```python
from build123d import *

# Parameters (mm, degrees)
SKETCH1_R                                      = 38.1
BOSS_EXTRUDE1_DEPTH                            = 6.35
CBORE_FOR_4_BUTTON_HEAD_CAP_SCREW1_D           = 2.8702
CBORE_FOR_4_BUTTON_HEAD_CAP_SCREW1_CBORE_D     = 4.826
CBORE_FOR_4_BUTTON_HEAD_CAP_SCREW1_CBORE_DEPTH = 1.905
CIRPATTERN1_COUNT                              = 8
SKETCH6_R                                      = 0.396875
CUT_EXTRUDE1_DEPTH                             = 55.254423783
CIRPATTERN2_COUNT                              = 4
SKETCH7_R                                      = 0.79375


with BuildPart() as part:
    # Sketch1 → Boss-Extrude1 (new body)
    with BuildSketch(Plane(origin=(0, 0, 0), x_dir=(1, 0, 0), z_dir=(0, 1, 0))):
        with Locations(Location((0, 0, 0), (0, 0, 270))):
            Circle(SKETCH1_R)
    extrude(amount=BOSS_EXTRUDE1_DEPTH)

    # CBORE for #4 Button Head Cap Screw1 (through all)
    with Locations(Plane(origin=(0, 0, 0), x_dir=(-1, 0, 0), z_dir=(0, -1, 0))):
        with Locations((0, -33.3375)):
            cbore_for_4_button_head_cap_screw1 = CounterBoreHole(CBORE_FOR_4_BUTTON_HEAD_CAP_SCREW1_D / 2, CBORE_FOR_4_BUTTON_HEAD_CAP_SCREW1_CBORE_D / 2, CBORE_FOR_4_BUTTON_HEAD_CAP_SCREW1_CBORE_DEPTH)

    # CirPattern1: CBORE for #4 Button Head Cap Screw1 ×8 about axis
    cirpattern1_axis = Axis((0, 0, 0), (0, 1, 0))
    for i in range(1, CIRPATTERN1_COUNT):
        add(cbore_for_4_button_head_cap_screw1.rotate(cirpattern1_axis, i * 360 / CIRPATTERN1_COUNT), mode=Mode.SUBTRACT)

    # Sketch6 → Cut-Extrude1 (cut, through all)
    with BuildSketch(Plane.XZ):
        with Locations(Location((-0.644070231, -1.381213067, 0), (0, 0, 270))):
            Circle(SKETCH6_R)
        with Locations(Location((-1.381213067, -0.644070231, 0), (0, 0, 270))):
            Circle(SKETCH6_R)
    cut_extrude1 = extrude(amount=-CUT_EXTRUDE1_DEPTH, mode=Mode.SUBTRACT)

    # CirPattern2: Cut-Extrude1 ×4 about axis
    cirpattern2_axis = Axis((0.000227094, 0, 0.000227094), (0, 1, 0))
    for i in range(1, CIRPATTERN2_COUNT):
        add(cut_extrude1.rotate(cirpattern2_axis, i * 360 / CIRPATTERN2_COUNT), mode=Mode.SUBTRACT)

    # Cut-Sweep1: sweep along a curve in space
    with BuildLine() as cut_sweep1_path:
        Line((0, 6.35, -8.001), (0, 0, -6.35))
    # Sketch7 → Cut-Sweep1 (sweep, cut)
    with BuildSketch(Plane(origin=(0, 6.35, 0), x_dir=(1, 0, 0), z_dir=(0, 1, 0))):
        with Locations((0, 8.001)):
            Circle(SKETCH7_R)
    sweep(path=cut_sweep1_path.line, mode=Mode.SUBTRACT)

    # CirPattern3: read off the stored shape, not the designer's step
    # CirPattern3: loft between two sections, ruled curve by curve
    cirpattern3_from = [
        Edge.make_bspline([(-7.470778066, 7.350046313, 0.003515494), (-7.470778066, 7.350046313, -1.583984506), (-9.058278066, 7.350046313, -1.583984506), (-9.058278066, 7.350046313, 0.003515494), (-9.058278066, 7.350046313, 1.591015494), (-7.470778066, 7.350046313, 1.591015494), (-7.470778066, 7.350046313, 0.003515494)], [0, 0, 0, 0, 0.5, 0.5, 0.5, 1, 1, 1, 1], 3, [1, 0.333333333, 0.333333333, 1, 0.333333333, 0.333333333, 1]),
    ]
    cirpattern3_to = [
        Edge.make_bspline([(-5.299753984, -1.000046313, 0.003515494), (-5.299753984, -1.000046313, -1.583984506), (-6.887253984, -1.000046313, -1.583984506), (-6.887253984, -1.000046313, 0.003515494), (-6.887253984, -1.000046313, 1.591015494), (-5.299753984, -1.000046313, 1.591015494), (-5.299753984, -1.000046313, 0.003515494)], [0, 0, 0, 0, 0.5, 0.5, 0.5, 1, 1, 1, 1], 3, [1, 0.333333333, 0.333333333, 1, 0.333333333, 0.333333333, 1]),
    ]
    cirpattern3 = Solid(Shell([*[Face.make_surface_from_curves(cirpattern3_from[k], cirpattern3_to[k]) for k in range(1)], Face(Wire(cirpattern3_from)), Face(Wire(cirpattern3_to))]))
    add(cirpattern3, mode=Mode.SUBTRACT)

    # CirPattern3 2: loft between two sections, ruled curve by curve
    cirpattern3_2_from = [
        Edge.make_bspline([(-5.31e-07, 7.350046313, 7.474293561), (-1.587500531, 7.350046313, 7.474293561), (-1.587500531, 7.350046313, 9.061793561), (-5.31e-07, 7.350046313, 9.061793561), (1.587499469, 7.350046313, 9.061793561), (1.587499469, 7.350046313, 7.474293561), (-5.31e-07, 7.350046313, 7.474293561)], [0, 0, 0, 0, 0.5, 0.5, 0.5, 1, 1, 1, 1], 3, [1, 0.333333333, 0.333333333, 1, 0.333333333, 0.333333333, 1]),
    ]
    cirpattern3_2_to = [
        Edge.make_bspline([(-5.31e-07, -1.000046313, 5.303269478), (-1.587500531, -1.000046313, 5.303269478), (-1.587500531, -1.000046313, 6.890769478), (-5.31e-07, -1.000046313, 6.890769478), (1.587499469, -1.000046313, 6.890769478), (1.587499469, -1.000046313, 5.303269478), (-5.31e-07, -1.000046313, 5.303269478)], [0, 0, 0, 0, 0.5, 0.5, 0.5, 1, 1, 1, 1], 3, [1, 0.333333333, 0.333333333, 1, 0.333333333, 0.333333333, 1]),
    ]
    cirpattern3_2 = Solid(Shell([*[Face.make_surface_from_curves(cirpattern3_2_from[k], cirpattern3_2_to[k]) for k in range(1)], Face(Wire(cirpattern3_2_from)), Face(Wire(cirpattern3_2_to))]))
    add(cirpattern3_2, mode=Mode.SUBTRACT)

    # CirPattern3 3: loft between two sections, ruled curve by curve
    cirpattern3_3_from = [
        Edge.make_bspline([(7.470777536, 7.350046313, 0.003516025), (7.470777536, 7.350046313, 1.591016025), (9.058277536, 7.350046313, 1.591016025), (9.058277536, 7.350046313, 0.003516025), (9.058277536, 7.350046313, -1.583983975), (7.470777536, 7.350046313, -1.583983975), (7.470777536, 7.350046313, 0.003516025)], [0, 0, 0, 0, 0.5, 0.5, 0.5, 1, 1, 1, 1], 3, [1, 0.333333333, 0.333333333, 1, 0.333333333, 0.333333333, 1]),
    ]
    cirpattern3_3_to = [
        Edge.make_bspline([(5.299753453, -1.000046313, 0.003516025), (5.299753453, -1.000046313, 1.591016025), (6.887253453, -1.000046313, 1.591016025), (6.887253453, -1.000046313, 0.003516025), (6.887253453, -1.000046313, -1.583983975), (5.299753453, -1.000046313, -1.583983975), (5.299753453, -1.000046313, 0.003516025)], [0, 0, 0, 0, 0.5, 0.5, 0.5, 1, 1, 1, 1], 3, [1, 0.333333333, 0.333333333, 1, 0.333333333, 0.333333333, 1]),
    ]
    cirpattern3_3 = Solid(Shell([*[Face.make_surface_from_curves(cirpattern3_3_from[k], cirpattern3_3_to[k]) for k in range(1)], Face(Wire(cirpattern3_3_from)), Face(Wire(cirpattern3_3_to))]))
    add(cirpattern3_3, mode=Mode.SUBTRACT)


solid = part.part
```
Input: part model. Units: mm. Frame: model coordinates. A direction names the side the tool comes from. Give positions to 0.01 mm unless a question says otherwise; leave off trailing zeros. Order: outer loops, then holes, each group sorted by start corner. A loop starts at its lowest first (then second) coordinate and runs counter-clockwise, first axis right, second up.
1. Cut plane C-C (y = 4.25). State how many separate pieces and enclosed holes the cut face has, and give its area (3 significant figures).
Computed:
separate pieces: 1
enclosed holes: 20
area: 4,500 mm2
2. Line query: probe 1 along Z at (x, y) = (1.5, 2.5); probe 2 along Z at (x, y) = (-32.5, 5.5); probe 3 along X at (y, z) = (4.25, 23.5). Output: solid intervals per line, ascending.
Computed:
probe 1: z = -38.07 to -1.02, -0.27 to 0.27, 1.02 to 38.07
probe 2: z = -19.88 to -1.17, 1.17 to 19.88
probe 3: x = -29.99 to -25.01, -22.14 to 22.14, 25.01 to 29.99
3. Cut plane B-B (z = 29.5). Return loops of the section in (x, y), and give its area (3 significant figures).
Computed:
outline: (-24.11, 0) - (24.11, 0) - (24.11, 6.35) - (-24.11, 6.35) - close
area: 306 mm2
4. Set-up query: faces 1 (the face through (-33, 1.905, -2)), 2 (the face through (34.74, 4.16, 0.31)). Return all of +Z, -Z, +X, -X, +Y, -Y with unobstructed straight access to the full face (end or side cutting, diameter ignored); none if empty.
Computed:
face 1: -Y
face 2: +Y, -Y
5. Pin query (flat end, axial travel): pin 1 Ø2.5 at (x, z) = (1, -33) entering from -Y (3 decimals); pin 2 Ø6 at (x, z) = (20.5, 2.5) entering from -Y; pin 3 Ø1.7 at (x, z) = (-23.57, 23.57) entering from -Y; pin 4 Ø2 at (x, y) = (26, 1.5) entering from +Z. Return the tip coordinate at first contact, or that it passes through.
Computed:
pin 1: stops at y = 1.905
pin 2: stops at y = 0
pin 3: passes through
pin 4: stops at z = 28.75
6. Draft query along X for faces 3 (the face through (2, 1.905, -33)), 4 (the face through (0.5, 0, -0.5)), 5 (the face through (-23.183, 3.131, -30.235)). Return one class per face: released by +X, released by -X, zero draft, split by the parting line, or undercut.
Computed:
face 3: undercut
face 4: zero draft
face 5: split by the parting line
7. Cut plane A-A (x = -15). Return loops of the section in (y, z), and give its area (3 significant figures).
Computed:
outline: (0, -35.02) - (6.35, -35.02) - (6.35, 35.02) - (0, 35.02) - close
area: 445 mm2
